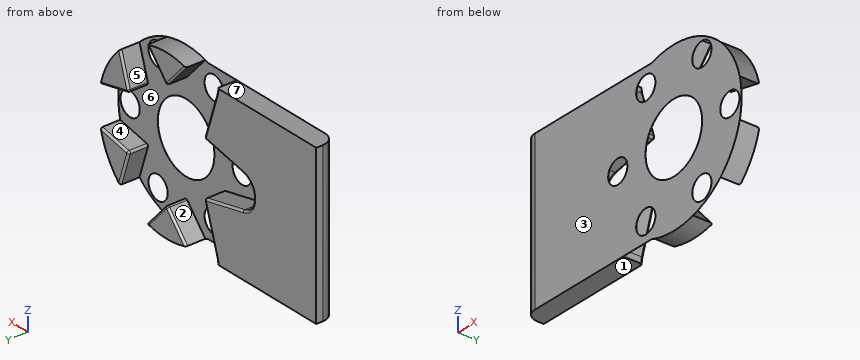
```python
from build123d import *

# Parameters (mm, degrees)
CROQUIS1_R              = 5.3
SALIENTE_EXTRUIR1_DEPTH = 3
CORTAR_EXTRUIR2_DEPTH   = 2.99
REDONDEO1_R             = 2
REDONDEO2_R             = 0.3
CROQUIS3_R              = 1.8
CORTAR_EXTRUIR3_DEPTH   = 10
MATRIZC1_COUNT          = 6


with BuildPart() as part:
    # Croquis1 → Saliente-Extruir1 (new body)
    with BuildSketch(Plane(origin=(0, 0, 0), x_dir=(1, 0, 0), z_dir=(0, 1, 0))):
        with BuildLine():
            Line((-28.04, 12), (-4.158124577, 12))
            ThreePointArc((-4.158124577, 12), (12.7, 0), (-4.158124577, -12))
            Line((-4.158124577, -12), (-28.04, -12))
            Line((-28.04, -12), (-28.04, 12))
        make_face()
        Circle(CROQUIS1_R, mode=Mode.SUBTRACT)
    extrude(amount=SALIENTE_EXTRUIR1_DEPTH)

    # Croquis2 → Cortar-Extruir2 (cut)
    with BuildSketch(Plane(origin=(0, 3, 0), x_dir=(1, 0, 0), z_dir=(0, 1, 0))):
        with BuildLine():
            Line((-14.335178977, -2.544323773), (-7.058107041, -4.075))
            Line((-7.058107041, -4.075), (-9.371038511, -11.142467275))
            ThreePointArc((-9.371038511, -11.142467275), (-8.2, -14.202816622), (-4.964140465, -13.686791048))
            Line((-4.964140465, -13.686791048), (0, -8.15))
            Line((0, -8.15), (4.964140465, -13.686791048))
            ThreePointArc((4.964140465, -13.686791048), (8.2, -14.202816622), (9.371038511, -11.142467275))
            Line((9.371038511, -11.142467275), (7.058107041, -4.075))
            Line((7.058107041, -4.075), (14.335178977, -2.544323773))
            ThreePointArc((14.335178977, -2.544323773), (16.4, 0), (14.335178977, 2.544323773))
            Line((14.335178977, 2.544323773), (7.058107041, 4.075))
            Line((7.058107041, 4.075), (9.371038511, 11.142467275))
            ThreePointArc((9.371038511, 11.142467275), (8.2, 14.202816622), (4.964140465, 13.686791048))
            Line((4.964140465, 13.686791048), (0, 8.15))
            Line((0, 8.15), (-4.964140465, 13.686791048))
            ThreePointArc((-4.964140465, 13.686791048), (-8.2, 14.202816622), (-9.371038511, 11.142467275))
            Line((-9.371038511, 11.142467275), (-7.058107041, 4.075))
            Line((-7.058107041, 4.075), (-14.335178977, 2.544323773))
            ThreePointArc((-14.335178977, 2.544323773), (-16.4, 0), (-14.335178977, -2.544323773))
        make_face()
    extrude(amount=-CORTAR_EXTRUIR2_DEPTH, mode=Mode.SUBTRACT)

    # Redondeo1
    redondeo1_edges = [part.edges().sort_by_distance(p)[0] for p in [
        (-28.04, 0, 0),
    ]]
    fillet(redondeo1_edges, radius=REDONDEO1_R)

    # Redondeo2
    redondeo2_edges = [part.edges().sort_by_distance(p)[0] for p in [
        (0, 1.505, -8.15),
        (7.058107041, 1.505, -4.075),
        (7.058107041, 1.505, 4.075),
        (0, 1.505, 8.15),
        (1.804886558, 3, 10.163093668),
        (7.899054019, 3, 6.644624444),
        (9.703940577, 3, 3.518469224),
        (9.703940577, 3, -3.518469224),
        (7.899054019, 3, -6.644624444),
        (1.804886558, 3, -10.163093668),
        (-1.804886558, 3, -10.163093668),
        (-9.471290512, 3, -11.565838876),
        (-8.214572776, 3, -7.608733638),
        (-10.696643009, 3, -3.309661887),
        (-16.4, 3, 0),
        (-10.696643009, 3, 3.309661887),
        (-8.214572776, 3, 7.608733638),
        (-9.471290512, 3, 11.565838876),
        (-1.804886558, 3, 10.163093668),
        (-7.058107041, 1.505, -4.075),
        (-7.058107041, 1.505, 4.075),
    ]]
    fillet(redondeo2_edges, radius=REDONDEO2_R)

    # Croquis3 → Cortar-Extruir3 (cut)
    with BuildSketch(Plane.XZ):
        with Locations((10.5, 0)):
            Circle(CROQUIS3_R)
    cortar_extruir3 = extrude(amount=-CORTAR_EXTRUIR3_DEPTH, mode=Mode.SUBTRACT)

    # MatrizC1: Cortar-Extruir3 ×6 about axis
    matrizc1_axis = Axis((0, 0, 0), (0, 1, 0))
    for i in range(1, MATRIZC1_COUNT):
        add(cortar_extruir3.rotate(matrizc1_axis, i * 360 / MATRIZC1_COUNT), mode=Mode.SUBTRACT)


solid = part.part
```
Input: part model. Units: mm. Frame: model coordinates. Face numbers are marked on the shaded views. A direction names the side the tool comes from. Give positions to 0.01 mm unless a question says otherwise; leave off trailing zeros. Loops run counter-clockwise (first coordinate to the right, second up) from the corner with the lowest first, then second, coordinate; pieces in that order, holes last.
1) Section query A-A on z = 0. Count the separate pieces of the cut face and the enclosed holes in it, and give its area (3 significant figures).
A:
separate pieces: 4
enclosed holes: 0
area: 34.2 mm2
2) Line query: L1, parallel to Z at x = 0, y = 0.05; L2, parallel to Z at x = -12.5, y = 2; L3, parallel to X at y = 0.45, z = 9. Output: solid intervals per line, ascending.
A:
L1: z = -12.7 to -8.3, 8.3 to 12.7
L2: z = -12 to -2.93, 2.93 to 12
L3: x = -27.3 to -8.67, -0.76 to 0.76, 8.67 to 8.96
3) Mould query, pull axis Z, two halves, no side actions, for the marked faces 1, 2, 3 and 4. Classes: released by +Z, released by -Z, zero draft, split by the parting line, or undercut.
A:
face 1: released by -Z
face 2: undercut
face 3: zero draft
face 4: undercut
4) Contact query for flat-ended pins moving along their axis: pin 1 (1 mm diameter, centred on y = 1, z = 1.5, fed in from -X); pin 2 (3 mm diameter, centred on x = -10.5, z = 0, fed in from +Y); pin 3 (4 mm diameter, centred on x = 5.25, z = -9.09, fed in from +Y); pin 4 (1.5 mm diameter, centred on x = -14.5, y = 1.5, fed in from -Z). Output: stop coordinate, or through.
A:
pin 1: stops at x = -27.98
pin 2: passes through
pin 3: stops at y = 0.01
pin 4: stops at z = -12
5) Section query B-B on y = 1.2. Return the cut outline in (x, z).
A:
outline: (-27.87, -12) - (-9.5, -12) arc R2.6 cw to (-9.37, -11.14) - (-7.16, -4.39) arc R0.3 ccw to (-7.39, -4.01) - (-14.34, -2.54) arc R2.6 cw to (-14.34, 2.54) - (-7.39, 4.01) arc R0.3 ccw to (-7.16, 4.39) - (-9.37, 11.14) arc R2.6 cw to (-9.5, 12) - (-27.87, 12) - close; (-3.61, -12.18) arc R12.7 ccw to (3.61, -12.18) - (0.22, -8.4) arc R0.3 ccw to (-0.22, -8.4) - close; (-3.61, 12.18) - (-0.22, 8.4) arc R0.3 ccw to (0.22, 8.4) - (3.61, 12.18) arc R12.7 ccw to start; (7.16, -4.39) - (8.74, -9.21) arc R12.7 ccw to (12.35, -2.96) - (7.39, -4.01) arc R0.3 ccw to start; (7.16, 4.39) arc R0.3 ccw to (7.39, 4.01) - (12.35, 2.96) arc R12.7 ccw to (8.74, 9.21) - close
6) Reachability of the marked faces 5, 6 and 7 from +Z, -Z, +X, -X, +Y, -Y: full face, straight path, thin tool, end or side. Return the list, or none.
A:
face 5: +Z, +Y
face 6: +Y
face 7: +Z, -X, +Y, -Y
7) Section query C-C on x = -20.5. Return the cut outline in (y, z), and give its area (3 significant figures).
A:
outline: (0, -12) - (3, -12) - (3, 12) - (0, 12) - close
area: 72.0 mm2
